CAD build for the part. Positions are in the model's coordinates, mm. Face numbers are marked on the shaded views. A direction names the side the tool comes from. Coordinates: 2 decimals unless noted, no trailing zeros. Loops run counter-clockwise (first coordinate to the right, second up) from the corner with the lowest first, then second, coordinate; pieces in that order, holes last. Notation, with made-up numbers: (-13.5, 27) -> (-5.5, 27) arc R16 cw to (-5.5, 51) -> close; hole circle Ø8 at (21.25, -32). An arc over 180 degrees is marked (long way). Answer as a JSON object with one key per item and string values. Group by question number.
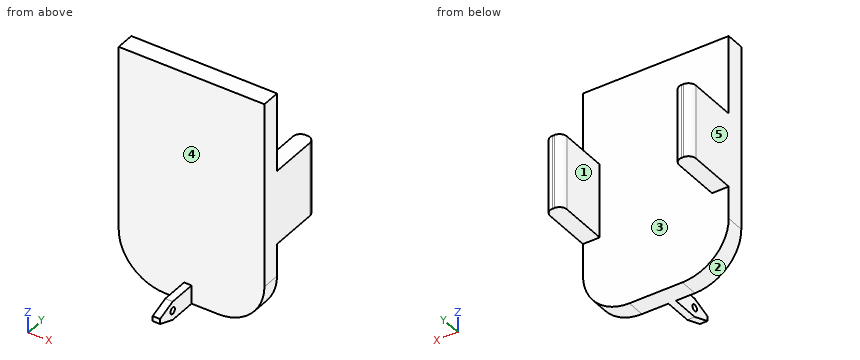
from build123d import *

# Parameters (mm, degrees)
BOSS_EXTRUDE2_DEPTH         = 5.08
SKETCH3_W                   = 4.572
SKETCH3_H                   = 20.32
BOSS_EXTRUDE3_DEPTH         = 15.24
FILLET1_R                   = 2.032
SKETCH4_W                   = 2.032
SKETCH4_H                   = 5.08
TILT_SERVO_CONNECTION_DEPTH = 12.7
SKETCH5_R                   = 0.889
CUT_EXTRUDE1_DEPTH          = 12.7
CHAMFER1_SIZE               = 5.08
CHAMFER1_SIZE2              = 1.84896879
CHAMFER1_PART_2_SIZE        = 5.08
CHAMFER1_PART_2_SIZE2       = 1.84896879


with BuildPart() as part:
    # Sketch1 → Boss-Extrude2 (new body)
    with BuildSketch(Plane(origin=(0, 0, 0), x_dir=(1, 0, 0), z_dir=(0, 1, 0))):
        with BuildLine():
            Line((-7.239, 31.75), (7.239, 31.75))
            ThreePointArc((7.239, 31.75), (16.219256121, 28.030256121), (19.939, 19.05))
            Line((19.939, 19.05), (19.939, -31.75))
            Line((19.939, -31.75), (-19.939, -31.75))
            Line((-19.939, -31.75), (-19.939, 19.05))
            ThreePointArc((-19.939, 19.05), (-16.219256121, 28.030256121), (-7.239, 31.75))
        make_face()
    extrude(amount=BOSS_EXTRUDE2_DEPTH)

    # Sketch3 → Boss-Extrude3 (add)
    with BuildSketch(Plane(origin=(0, 5.08, 0), x_dir=(1, 0, 0), z_dir=(0, 1, 0))):
        with Locations((-17.653, 0)):
            Rectangle(SKETCH3_W, SKETCH3_H)
        with Locations((17.653, 0)):
            Rectangle(SKETCH3_W, SKETCH3_H)
    extrude(amount=BOSS_EXTRUDE3_DEPTH)

    # Fillet1
    fillet1_edges = [part.edges().sort_by_distance(p)[0] for p in [
        (-19.939, 20.32, 0),
        (-15.367, 20.32, 0),
        (19.939, 20.32, 0),
        (15.367, 20.32, 0),
    ]]
    fillet(fillet1_edges, radius=FILLET1_R)

    # Sketch4 → Tilt servo connection (add)
    with BuildSketch(Plane.XZ):
        with Locations((-1.016, -29.21)):
            Rectangle(SKETCH4_W, SKETCH4_H)
    extrude(amount=TILT_SERVO_CONNECTION_DEPTH)

    # Sketch5 → Cut-Extrude1 (cut)
    with BuildSketch(Plane(origin=(0, 0, 0), x_dir=(0, 0, -1), z_dir=(1, 0, 0))):
        with Locations((29.21, -7.62)):
            Circle(SKETCH5_R)
    extrude(amount=-CUT_EXTRUDE1_DEPTH, mode=Mode.SUBTRACT)

    # Chamfer1
    chamfer1_edges = [part.edges().sort_by_distance(p)[0] for p in [
        (-1.016, -12.7, -31.75),
    ]]
    chamfer1_side = [part.faces().sort_by_distance(p)[0] for p in [
        (-0.263896104, 0.230909091, -31.75),
    ]]
    chamfer(chamfer1_edges, length=CHAMFER1_SIZE, length2=CHAMFER1_SIZE2, reference=chamfer1_side[0])

    # Chamfer1 part 2
    chamfer1_part_2_edges = [part.edges().sort_by_distance(p)[0] for p in [
        (-1.016, -12.7, -26.67),
    ]]
    chamfer1_part_2_side = [part.faces().sort_by_distance(p)[0] for p in [
        (-1.016, -6.35, -26.67),
    ]]
    chamfer(chamfer1_part_2_edges, length=CHAMFER1_PART_2_SIZE, length2=CHAMFER1_PART_2_SIZE2, reference=chamfer1_part_2_side[0])


solid = part.part
Item 1: Band-saw the part on C-C, the plane z = -29.21. List the corners of the cut face in (x, y), and give its area (3 significant figures).
Item 2: Band-saw the part on B-B, the plane z = -2. List the corners of the cut face in (x, y).
Item 3: Band-saw the part on D-D, the plane x = -16.5. List the corners of the cut face in (y, z), and give its area (3 significant figures).
Item 4: Drill centre lines: L1, parallel to Y at x = -0.45, z = -29.21; L2, parallel to X at y = 14.5, z = -10; L3, parallel to Y at x = 10.5, z = -9. Where is each one in solid material? Low to high.
Item 5: Flat gauge pins, fed straight in: P1, Ø3.5, axis at x = 18, y = 10, coming from the -Z side; P2, Ø1.5, axis at y = -5, z = -28, coming from the -X side; P3, Ø1, axis at x = 4, z = 7, coming from the +Y side. Where does each tip first touch, or does it go through?
Item 6: 3-axis set-ups, long thin cutter, end or side, ignore diameter. For the marked faces 1 and 2: which of +Z, -Z, +X, -X, +Y, -Y reach the whole face in a straight line?
Item 7: Band-saw the part on A-A, the plane y = 6. List the corners of the cut face in (x, z).
Item 8: Pull direction X, two halves, no side cores. Call the marked faces 3, 4 and 5: +X half, -X half, draft (parallel to the pull), parting line (faces both ways), or undercut.
Reply:
{
 "1": {"outline": "(-14.86, 0) -> (-2.03, 0) -> (-2.03, -6.73) -> (0, -6.73) -> (0, 0) -> (14.86, 0) -> (14.86, 5.08) -> (-14.86, 5.08) -> close; (-2.03, -12.7) -> (0, -12.7) -> (0, -8.51) -> (-2.03, -8.51) -> close", "area": "173 mm²"},
 "2": {"outline": "(-19.94, 0) -> (19.94, 0) -> (19.94, 18.29) arc R2.03 ccw to (17.91, 20.32) -> (17.4, 20.32) arc R2.03 ccw to (15.37, 18.29) -> (15.37, 5.08) -> (-15.37, 5.08) -> (-15.37, 18.29) arc R2.03 ccw to (-17.4, 20.32) -> (-17.91, 20.32) arc R2.03 ccw to (-19.94, 18.29) -> close"},
 "3": {"outline": "(0, -27.74) -> (5.08, -27.74) -> (5.08, -10.16) -> (20.11, -10.16) -> (20.11, 10.16) -> (5.08, 10.16) -> (5.08, 31.75) -> (0, 31.75) -> close", "area": "608 mm²"},
 "4": {"L1": "-12.7 to -8.51, -6.73 to 5.08", "L2": "-19.94 to -15.37, 15.37 to 19.94", "L3": "0 to 5.08"},
 "5": {"P1": "z = -10.16", "P2": "x = -2.03", "P3": "y = 5.08"},
 "6": {"face 1": "+Z, -Z, +Y", "face 2": "-Z, -X, +Y, -Y"},
 "7": {"outline": "(-19.94, -10.16) -> (-15.37, -10.16) -> (-15.37, 10.16) -> (-19.94, 10.16) -> close; (15.37, -10.16) -> (19.94, -10.16) -> (19.94, 10.16) -> (15.37, 10.16) -> close"},
 "8": {"face 3": "undercut", "face 4": "draft", "face 5": "-X half"}
}
